```python
from build123d import *

# Parameters (mm, degrees)
SKETCH1_W               = 76.2
SKETCH1_H               = 50.8
BOSS_EXTRUDE1_DEPTH     = 12.7
F_1_4_20_TAPPED_HOLE1_D = 5.1054


with BuildPart() as part:
    # Sketch1 → Boss-Extrude1 (new body)
    with BuildSketch(Plane(origin=(0, 0, 0), x_dir=(1, 0, 0), z_dir=(0, 1, 0))):
        Rectangle(SKETCH1_W, SKETCH1_H)
    extrude(amount=BOSS_EXTRUDE1_DEPTH)

    # 1/4-20 Tapped Hole1 (through all)
    with Locations(Plane(origin=(0, 12.7, 0), x_dir=(1, 0, 0), z_dir=(0, 1, 0))):
        with Locations((-31.75, 0), (31.75, 0)):
            Hole(F_1_4_20_TAPPED_HOLE1_D / 2)


solid = part.part
```
For this review, take the finished solid that the model builds, in its own axes (mm). Round coordinates to 2 decimals unless told otherwise and drop trailing zeros. Loops run counter-clockwise (first coordinate to the right, second up) from the corner with the lowest first, then second, coordinate; pieces in that order, holes last.
(1) We need section A-A (x = -31.75). Give the boundary of the cut face in (y, z).
Returned:
outline: (0, -25.4) - (12.7, -25.4) - (12.7, -2.55) - (0, -2.55) - close; (0, 2.55) - (12.7, 2.55) - (12.7, 25.4) - (0, 25.4) - close
(2) Mouldability with a two-part tool opening along X and no side actions: class faces 1 (the cylindrical face through (-34.185, 6.261, -0.767)), 2 (the flat face through (38.1, 6, 0)), 3 (the flat face through (-1, 6, -25.4)) as released by +X, released by -X, zero draft, split by the parting line, or undercut.
Returned:
face 1: undercut
face 2: released by +X
face 3: zero draft
(3) Clearance check with a flat-ended pin moving along its axis: P1, Ø4, axis at x = -31.75, z = 0, coming from the -Y side. State where the tip first meets the part, or that it passes through.
Returned:
P1: passes through
(4) We need section B-B (z = 0). Give the boundary of the cut face in (x, y), plus the area to 3 significant figures.
Returned:
outline: (-38.1, 0) - (-34.3, 0) - (-34.3, 12.7) - (-38.1, 12.7) - close; (-29.2, 0) - (29.2, 0) - (29.2, 12.7) - (-29.2, 12.7) - close; (34.3, 0) - (38.1, 0) - (38.1, 12.7) - (34.3, 12.7) - close
area: 838 mm2
(5) Wall thickness on line 1 along Z through (x, y) = (31.75, 3.5); line 2 along X through (y, z) = (2.5, 1); line 3 along X through (y, z) = (6, 2): over which ranges is each line inside the solid? List them lowest first.
Returned:
line 1: z = -25.4 to -2.55, 2.55 to 25.4
line 2: x = -38.1 to -34.1, -29.4 to 29.4, 34.1 to 38.1
line 3: x = -38.1 to -33.34, -30.16 to 30.16, 33.34 to 38.1
